from build123d import *

# Parameters (mm, degrees)
SKETCH_1_W          = 16.1
SKETCH_1_H          = 16.1
EXTRUDE_1_DEPTH     = 0.2
SKETCH_2_W          = 16.5
SKETCH_2_H          = 16.5
SKETCH_2_W_2        = 16.1
SKETCH_2_H_2        = 16.1
EXTRUDE_2_DEPTH     = 3.61
FILLET_1_R          = 0.2
SKETCH_3_W          = 0.2
SKETCH_3_H          = 3
SKETCH_3_W_2        = 3
SKETCH_3_H_2        = 0.2
CUT_EXTRUDE_1_DEPTH = 0.51


with BuildPart() as part:
    # 草图1 → 凸台-拉伸1 (new body)
    with BuildSketch(Plane(origin=(0, 0, 0), x_dir=(1, 0, 0), z_dir=(0, 1, 0))):
        with Locations((8.25, -8.25)):
            Rectangle(SKETCH_1_W, SKETCH_1_H)
        with BuildLine():
            Line((1.706516818, -15.5), (1, -14.793483182))
            Line((1, -14.793483182), (1, -8.75))
            ThreePointArc((1, -8.75), (1.24, -8.51), (1.48, -8.75))
            Line((1.48, -8.75), (5.291960108, -8.75))
            ThreePointArc((5.291960108, -8.75), (6.128679656, -10.371320344), (7.75, -11.208039892))
            Line((7.75, -11.208039892), (7.75, -15.02))
            ThreePointArc((7.75, -15.02), (7.99, -15.26), (7.75, -15.5))
            Line((7.75, -15.5), (1.706516818, -15.5))
        make_face(mode=Mode.SUBTRACT)
        with BuildLine():
            Line((5.291960108, -7.75), (1.48, -7.75))
            ThreePointArc((1.48, -7.75), (1.24, -7.99), (1, -7.75))
            Line((1, -7.75), (1, -1.706516818))
            Line((1, -1.706516818), (1.706516818, -1))
            Line((1.706516818, -1), (7.75, -1))
            ThreePointArc((7.75, -1), (7.99, -1.24), (7.75, -1.48))
            Line((7.75, -1.48), (7.75, -5.291960108))
            ThreePointArc((7.75, -5.291960108), (6.128679656, -6.128679656), (5.291960108, -7.75))
        make_face(mode=Mode.SUBTRACT)
        with BuildLine():
            Line((8.75, -1), (14.793483182, -1))
            Line((14.793483182, -1), (15.5, -1.706516818))
            Line((15.5, -1.706516818), (15.5, -7.75))
            ThreePointArc((15.5, -7.75), (15.26, -7.99), (15.02, -7.75))
            Line((15.02, -7.75), (11.208039892, -7.75))
            ThreePointArc((11.208039892, -7.75), (10.371320344, -6.128679656), (8.75, -5.291960108))
            Line((8.75, -5.291960108), (8.75, -1.48))
            ThreePointArc((8.75, -1.48), (8.51, -1.24), (8.75, -1))
        make_face(mode=Mode.SUBTRACT)
        with BuildLine():
            Line((15.5, -8.75), (15.5, -14.793483182))
            Line((15.5, -14.793483182), (14.793483182, -15.5))
            Line((14.793483182, -15.5), (8.75, -15.5))
            ThreePointArc((8.75, -15.5), (8.51, -15.26), (8.75, -15.02))
            Line((8.75, -15.02), (8.75, -11.208039892))
            ThreePointArc((8.75, -11.208039892), (10.371320344, -10.371320344), (11.208039892, -8.75))
            Line((11.208039892, -8.75), (15.02, -8.75))
            ThreePointArc((15.02, -8.75), (15.26, -8.51), (15.5, -8.75))
        make_face(mode=Mode.SUBTRACT)
    extrude(amount=-EXTRUDE_1_DEPTH)

    # 草图2 → 凸台-拉伸2 (add)
    with BuildSketch(Plane(origin=(0, 0, 0), x_dir=(1, 0, 0), z_dir=(0, 1, 0))):
        with Locations((8.25, -8.25)):
            Rectangle(SKETCH_2_W, SKETCH_2_H)
        with Locations((8.25, -8.25)):
            Rectangle(SKETCH_2_W_2, SKETCH_2_H_2, mode=Mode.SUBTRACT)
    extrude(amount=-EXTRUDE_2_DEPTH)

    # 圆角1
    fillet_1_edges = [part.edges().sort_by_distance(p)[0] for p in [
        (16.5, 0, 8.25),
        (8.25, 0, 0),
        (0, 0, 8.25),
        (8.25, 0, 16.5),
    ]]
    fillet(fillet_1_edges, radius=FILLET_1_R)

    # 草图3 → 切除-拉伸1 (cut)
    with BuildSketch(Plane.XZ.offset(3.61)):
        with Locations((0.1, 11.24)):
            Rectangle(SKETCH_3_W, SKETCH_3_H)
        with Locations((0.1, 5.24)):
            Rectangle(SKETCH_3_W, SKETCH_3_H)
        with Locations((16.4, 11.24)):
            Rectangle(SKETCH_3_W, SKETCH_3_H)
        with Locations((16.4, 5.24)):
            Rectangle(SKETCH_3_W, SKETCH_3_H)
        with Locations((5.26, 16.4)):
            Rectangle(SKETCH_3_W_2, SKETCH_3_H_2)
        with Locations((11.26, 16.4)):
            Rectangle(SKETCH_3_W_2, SKETCH_3_H_2)
        with Locations((11.26, 0.1)):
            Rectangle(SKETCH_3_W_2, SKETCH_3_H_2)
        with Locations((5.26, 0.1)):
            Rectangle(SKETCH_3_W_2, SKETCH_3_H_2)
    extrude(amount=-CUT_EXTRUDE_1_DEPTH, mode=Mode.SUBTRACT)


solid = part.part
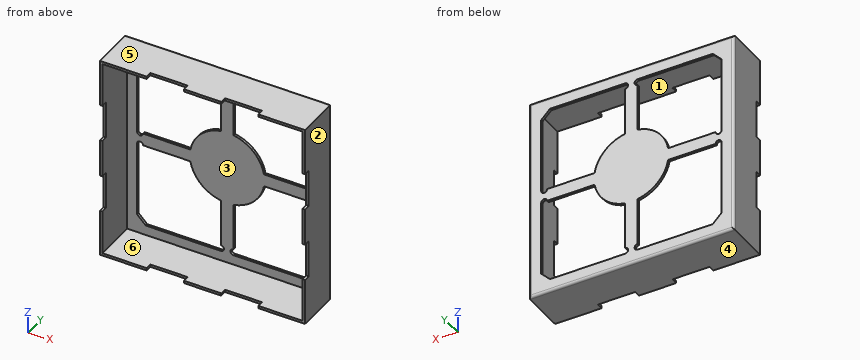
Verification items for the finished model (mm, model axes). Face numbers are marked on the shaded views. A direction names the side the tool comes from. Coordinates: 2 decimals unless noted, no trailing zeros. Order: outer loops, then holes, each group sorted by start corner. A loop starts at its lowest first (then second) coordinate and runs counter-clockwise, first axis right, second up. Notation, with made-up numbers: (-15.5, -34.5) -> (2.5, -34.5) arc R36 cw to (2.5, -0.5) -> close; hole circle Ø3 at (5, -23.5). An arc over 180 degrees is marked (long way). Put each result on its own line as item: value. Start each with the question number.
1. Go/stop test with a flat-tipped pin: pin 1 Ø8 at (x, z) = (12, 7.5) entering from +Y. Record where the tip stops, or that it passes through.
2. Cross-section at B-B, the plane z = 12.5. Record the boundary of the cut face in (x, y).
3. Material ranges on L1, parallel to Z at x = 15, y = -0.65; L2, parallel to X at y = -0.15, z = 3.75, recorded low to high. Write a range as [from, to].
4. Cross-section at A-A, the plane x = 13.75. Record the boundary of the cut face in (y, z).
5. Access from +Z, -Z, +X, -X, +Y, -Y to the whole of each face (thin tool, end or side, straight path). Record for the marked faces 5 and 6.
6. Mould release check, pull along X, two halves, no side actions. Record for the marked faces 1, 2, 3 and 4: released by +X, released by -X, zero draft, split by the parting line, or undercut.
Computed:
1. pin 1: y = 0
2. outline: (0, -3.1) -> (0.2, -3.1) -> (0.2, -0.2) -> (1, -0.2) -> (1, 0) -> (0.2, 0) arc R0.2 ccw to (0, -0.2) -> close; (7.75, -0.2) -> (8.75, -0.2) -> (8.75, 0) -> (7.75, 0) -> close; (15.5, -0.2) -> (16.3, -0.2) -> (16.3, -3.1) -> (16.5, -3.1) -> (16.5, -0.2) arc R0.2 ccw to (16.3, 0) -> (15.5, 0) -> close
3. L1: [0, 0.2], [16.3, 16.5]
3. L2: [0.01, 1], [7.75, 8.75], [15.5, 16.49]
4. outline: (-3.61, 0) -> (-0.2, 0) arc R0.2 ccw to (0, 0.2) -> (0, 1) -> (-0.2, 1) -> (-0.2, 0.2) -> (-3.61, 0.2) -> close; (-3.61, 16.3) -> (-0.2, 16.3) -> (-0.2, 15.5) -> (0, 15.5) -> (0, 16.3) arc R0.2 ccw to (-0.2, 16.5) -> (-3.61, 16.5) -> close; (-0.2, 7.75) -> (0, 7.75) -> (0, 8.75) -> (-0.2, 8.75) -> close
5. face 5: +Z, +X, -X, +Y, -Y
5. face 6: -Y
6. face 1: undercut
6. face 2: released by +X
6. face 3: undercut
6. face 4: zero draft
